The listing builds one solid part. Answer for the finished solid, in the listing's coordinates (mm). A direction names the side the tool comes from. Coordinates: 2 decimals unless noted, no trailing zeros. Loops run counter-clockwise (first coordinate to the right, second up) from the corner with the lowest first, then second, coordinate; pieces in that order, holes last. Notation, with made-up numbers: (30, -31.5) - (35, -31.5) arc R22 cw to (35, -2.5) - close; hole circle Ø1 at (79.5, -18.5). An arc over 180 degrees is marked (long way). Return JSON: item names as keys, results as strings. Group by question number.
1. Find the intervals of material crossed by line 1 along X through (y, z) = (48.26, 14.5); line 2 along X through (y, z) = (15.5, 8), in increasing order.
2. Section B-B (z = 13.75) is taken. Write down the section's boundary in (x, y) (3 decimals).
3. Which of the six approach directions +Z, -Z, +X, -X, +Y, -Y give full straight-line access (tool end or side, diameter ignored) to faces 1 (the face through (7.62, 25, 6)), 2 (the face through (48.16, 46.4, 10.3))?
4. This flat-tipped pin is pushed along its axis until it touches: P1, Ø3, axis at x = 34, y = 41, coming from the -Z side. Where does it stop, or does it pass through?
5. Section D-D (x = 36) is taken. Write down the section's boundary in (y, z).
6. Section C-C (x = 18) is taken. Write down the section's boundary in (y, z).
7. The mould has two halves that part along Y. Classify faces 3 (the face through (3.71, 46.4, 10.3)), 4 (the face through (6, 26, 0)), 5 (the face through (25, 50.8, 10)): pulls with the +Y half, pulls with the -Y half, needs draft (parallel to the pull), parting line crosses it, or undercut.
8. Section A-A (y = 48.26) is taken. Write down the section's boundary in (x, z), and give its area (3 significant figures).
```python
from build123d import *

# Parameters (mm, degrees)
SKETCH7_W               = 50.8
SKETCH7_H               = 50.8
BOSS_EXTRUDE3_DEPTH     = 20.32
SHELL4_T                = -7.62
CUT_EXTRUDE4_DEPTH      = 20.066
CUT_EXTRUDE4_DEPTH_BACK = 73.955945611
SKETCH10_R              = 1.905
SKETCH11_R              = 4.7879
CUT_EXTRUDE5_DEPTH      = 7.62


with BuildPart() as part:
    # Sketch7 → Boss-Extrude3 (new body)
    with BuildSketch(Plane.XY):
        with Locations((25.4, 25.4)):
            Rectangle(SKETCH7_W, SKETCH7_H)
    extrude(amount=BOSS_EXTRUDE3_DEPTH)

    # Shell4
    shell4_openings = [part.faces().sort_by_distance(p)[0] for p in [
        (25.4, 25.4, 0),
    ]]
    offset(amount=SHELL4_T, openings=shell4_openings, kind=Kind.INTERSECTION)

    # Sketch10 → Cut-Extrude4 (cut, two sides: drawn at the far end of the back side and taken through both)
    with BuildSketch(Plane(origin=(0, 0, 12.7), x_dir=(-1, 0, 0), z_dir=(0, 0, -1)).offset(-CUT_EXTRUDE4_DEPTH_BACK)):
        with Locations((-47.752, 48.26)):
            Circle(SKETCH10_R)
        with Locations((-3.302, 48.26)):
            Circle(SKETCH10_R)
        with Locations((-47.752, 2.54)):
            Circle(SKETCH10_R)
        with Locations((-3.302, 3.81)):
            Circle(SKETCH10_R)
    extrude(amount=CUT_EXTRUDE4_DEPTH + CUT_EXTRUDE4_DEPTH_BACK, mode=Mode.SUBTRACT)

    # Sketch11 → Cut-Extrude5 (cut)
    with BuildSketch(Plane(origin=(0, 0, 12.7), x_dir=(-1, 0, 0), z_dir=(0, 0, -1))):
        with Locations((-21.082, 22.86)):
            Circle(SKETCH11_R)
    extrude(amount=-CUT_EXTRUDE5_DEPTH, mode=Mode.SUBTRACT)


solid = part.part
```
The answers:
{
 "1": {"line 1": "x = 0 to 1.4, 5.21 to 45.85, 49.66 to 50.8", "line 2": "x = 0 to 7.62, 43.18 to 50.8"},
 "2": {"outline": "(0, 0) - (50.8, 0) - (50.8, 50.8) - (0, 50.8) - close; hole circle Ø3.81 at (3.302, 3.81); hole circle Ø3.81 at (3.302, 48.26); hole circle Ø9.576 at (21.082, 22.86); hole circle Ø3.81 at (47.752, 2.54); hole circle Ø3.81 at (47.752, 48.26)"},
 "3": {"face 1": "-Z", "face 2": "+Z, -Z"},
 "4": {"P1": "stops at z = 12.7"},
 "5": {"outline": "(0, 0) - (7.62, 0) - (7.62, 12.7) - (43.18, 12.7) - (43.18, 0) - (50.8, 0) - (50.8, 20.32) - (0, 20.32) - close"},
 "6": {"outline": "(0, 0) - (7.62, 0) - (7.62, 12.7) - (19.2, 12.7) - (19.2, 20.32) - (0, 20.32) - close; (26.52, 12.7) - (43.18, 12.7) - (43.18, 0) - (50.8, 0) - (50.8, 20.32) - (26.52, 20.32) - close"},
 "7": {"face 3": "undercut", "face 4": "needs draft", "face 5": "pulls with the +Y half"},
 "8": {"outline": "(0, 0) - (1.4, 0) - (1.4, 20.32) - (0, 20.32) - close; (5.21, 0) - (45.85, 0) - (45.85, 20.32) - (5.21, 20.32) - close; (49.66, 0) - (50.8, 0) - (50.8, 20.32) - (49.66, 20.32) - close", "area": "877 mm2"}
}
